Print and shaded views of the part. All mm, measured from the part's lowest x, y and z. A direction names the side the tool comes from. Round coordinates to 2 decimals unless told otherwise and drop trailing zeros. Loops run counter-clockwise (first coordinate to the right, second up) from the corner with the lowest first, then second, coordinate; pieces in that order, holes last. Notation, with made-up numbers: (-7.5, 3.25) - (49.5, 3.25) arc R15 ccw to (49.5, 22.25) - close; hole circle Ø5 at (24, 88.5). An arc over 180 degrees is marked (long way). Use one line per item in the form item = value.
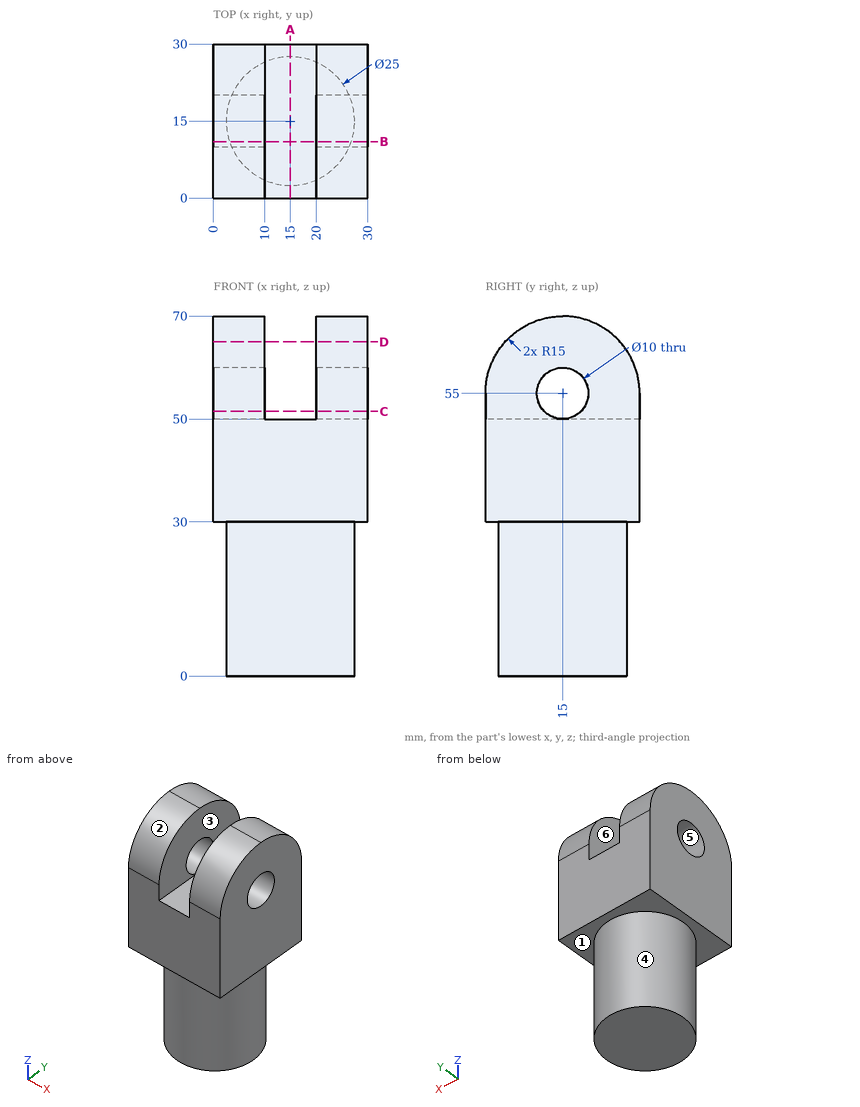
1) Slice it at C-C (z = 51.5). Write the cut outline in (x, y), plus the area to 3 significant figures.
Report:
outline = (0, 0) - (10, 0) - (10, 11.43) - (0, 11.43) - close; (0, 18.57) - (10, 18.57) - (10, 30) - (0, 30) - close; (20, 0) - (30, 0) - (30, 11.43) - (20, 11.43) - close; (20, 18.57) - (30, 18.57) - (30, 30) - (20, 30) - close
area = 457 mm^2
2) Drill centre lines: probe 1 along Y at (x, z) = (7.25, 55); probe 2 along Z at (x, y) = (7.5, 15). Where is each one in solid material? Low to high.
Report:
probe_1 = 0 to 10, 20 to 30
probe_2 = 0 to 50, 60 to 70
3) Slice it at A-A (x = 15). Write the cut outline in (y, z), plus the area to 3 significant figures.
Report:
outline = (0, 30) - (2.5, 30) - (2.5, 0) - (27.5, 0) - (27.5, 30) - (30, 30) - (30, 50) - (0, 50) - close
area = 1,350 mm^2
4) Slice it at D-D (z = 65). Write the cut outline in (x, y).
Report:
outline = (0, 3.82) - (10, 3.82) - (10, 26.18) - (0, 26.18) - close; (20, 3.82) - (30, 3.82) - (30, 26.18) - (20, 26.18) - close
5) Flat gauge pins, fed straight in: pin 1 (5 mm diameter, centred on x = 4.5, z = 16.5, fed in from +Y) (1 decimal); pin 2 (8 mm diameter, centred on y = 15, z = 55, fed in from +X); pin 3 (4 mm diameter, centred on y = 24.5, z = 16, fed in from +X); pin 4 (1 mm diameter, centred on x = 9.5, y = 7, fed in from +Z). Where does each tip first touch, or does it go through?
Report:
pin_1 = 24.6
pin_2 = through
pin_3 = 25
pin_4 = 67.99
6) Two-plate mould, pull along Y, no slides. Class the marked faces 4, 5 and 6: +Y half, -Y half, draft (parallel to the pull), parting line (faces both ways), or undercut.
Report:
face_4 = parting line
face_5 = undercut
face_6 = draft
7) Slice it at B-B (y = 11). Write the cut outline in (x, z).
Report:
outline = (0, 30) - (3.16, 30) - (3.16, 0) - (26.84, 0) - (26.84, 30) - (30, 30) - (30, 52) - (20, 52) - (20, 50) - (10, 50) - (10, 52) - (0, 52) - close; (0, 58) - (10, 58) - (10, 69.46) - (0, 69.46) - close; (20, 58) - (30, 58) - (30, 69.46) - (20, 69.46) - close
8) Tool access for the marked faces 1, 2 and 3: list every direction of +Z, -Z, +X, -X, +Y, -Y with a clear straight run to the whole face (end or side of a thin tool).
Report:
face_1 = -Z
face_2 = +Z, +X, -X, -Y
face_3 = +Z, +Y, -Y
